Answer from the drawing. Dimensions are ordinates in mm from the lowest x, y and z of the part. Round coordinates to 2 decimals unless told otherwise and drop trailing zeros. Loops run counter-clockwise (first coordinate to the right, second up) from the corner with the lowest first, then second, coordinate; pieces in that order, holes last.
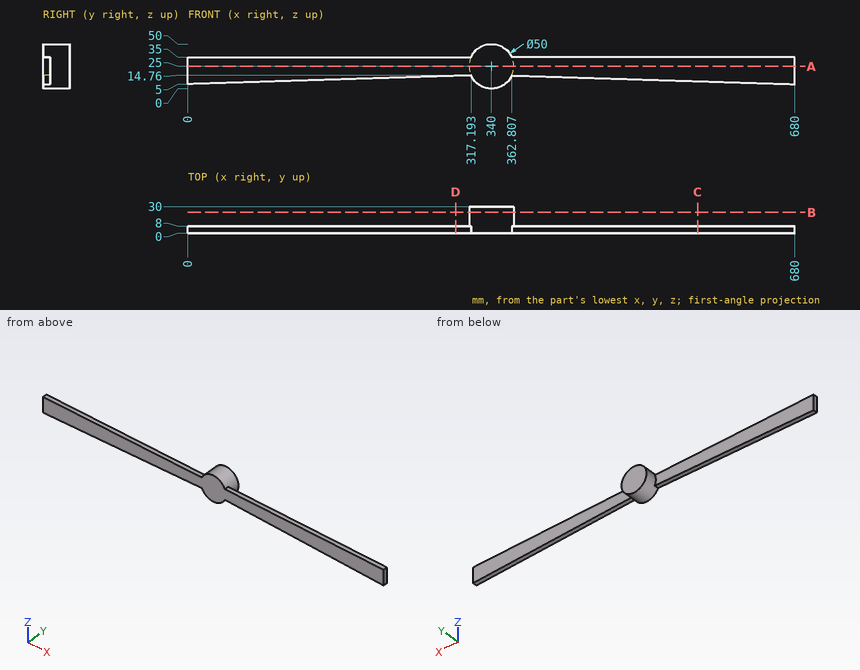
1. Find section D-D (x = 300). Write down the section's boundary in (y, z).
Answer key:
outline: (0, 14.23) - (8, 14.23) - (8, 35) - (0, 35) - close
2. Given pin 1 (1 mm diameter, centred on x = 314, y = 23.5, fed in from -Z); pin 2 (2.5 mm diameter, centred on x = 553, y = 5.5, fed in from +Z); pin 3 (12 mm diameter, centred on x = 294.5, z = 12.5, fed in from +Y); pin 4 (1 mm diameter, centred on y = 15, z = 35, fed in from -X) (1 decimal), each flat-ended and moving along its own axis, determine where each tip first touches the part or whether it passes through.
Answer key:
pin 1: passes through
pin 2: stops at z = 35
pin 3: stops at y = 8
pin 4: stops at x = 316.9
3. Find section A-A (z = 25). Write down the section's boundary in (x, y).
Answer key:
outline: (0, 0) - (680, 0) - (680, 8) - (365, 8) - (365, 30) - (315, 30) - (315, 8) - (0, 8) - close
4. Find section B-B (y = 23.5). Write down the section's boundary in (x, z), then the cut area to 3 significant figures.
Answer key:
outline: circle Ø50 at (340, 25)
area: 1,960 mm2
5. Consider probe 1 along Y at (x, z) = (404.5, 21); probe 2 along X at (y, z) = (27.5, 23); probe 3 along X at (y, z) = (9.5, 39). Determine where each line is inside the solid, lowest interval first.
Answer key:
probe 1: y = 0 to 8
probe 2: x = 315.08 to 364.92
probe 3: x = 319.29 to 360.71
6. Find section C-C (x = 571). Write down the section's boundary in (y, z).
Answer key:
outline: (0, 8.35) - (8, 8.35) - (8, 35) - (0, 35) - close
